```python
from build123d import *

# Parameters (mm, degrees)
SKETCH2_R           = 4
CUT_EXTRUDE1_DEPTH  = 0.5
SKETCH3_R           = 2.2
BOSS_EXTRUDE1_DEPTH = 0.5
SKETCH4_R           = 1.55
CUT_EXTRUDE2_DEPTH  = 16.305227865
CHAMFER1_SIZE       = 0.25


with BuildPart() as part:
    # Sketch1 → Revolve1 (revolve)
    with BuildSketch(Plane.XY, mode=Mode.PRIVATE) as revolve1_sk:
        Polygon((0, 0), (-9, 0), (-9, 1), (-6, 1), (-6, 7.5), (-9, 7.5), (-9, 8.5), (0, 8.5), align=None)
    revolve(revolve1_sk.sketch.rotate(Axis((0, 8.5, 0), (0, -1, 0)), 270), axis=Axis((0, 8.5, 0), (0, -1, 0)))

    # Sketch2 → Cut-Extrude1 (cut)
    with BuildSketch(Plane.XZ):
        with Locations(Location((0, 0, 0), (0, 0, 270))):
            Circle(SKETCH2_R)
    cut_extrude1 = extrude(amount=-CUT_EXTRUDE1_DEPTH, mode=Mode.SUBTRACT)

    # Sketch3 → Boss-Extrude1 (add)
    with BuildSketch(Plane.XZ.offset(-0.5)):
        with Locations(Location((0, 0, 0), (0, 0, 270))):
            Circle(SKETCH3_R)
    boss_extrude1 = extrude(amount=BOSS_EXTRUDE1_DEPTH)

    # Mirror1: Cut-Extrude1, Boss-Extrude1 across plane
    add(cut_extrude1.mirror(Plane.ZX.offset(4.25)), mode=Mode.SUBTRACT)
    add(boss_extrude1.mirror(Plane.ZX.offset(4.25)))

    # Sketch4 → Cut-Extrude2 (cut, through all)
    with BuildSketch(Plane.XZ):
        with Locations(Location((0, 0, 0), (0, 0, 270))):
            Circle(SKETCH4_R)
    extrude(amount=-CUT_EXTRUDE2_DEPTH, mode=Mode.SUBTRACT)

    # Chamfer1
    chamfer1_edges = [part.edges().sort_by_distance(p)[0] for p in [
        (0, 8.5, -9),
        (0, 7.5, -6),
        (0, 1, -6),
        (0, 0, -9),
    ]]
    chamfer(chamfer1_edges, length=CHAMFER1_SIZE)


solid = part.part
```
Work out the finished part from the listing and answer in its coordinate system (mm). A direction names the side the tool comes from. Coordinates: 2 decimals unless noted, no trailing zeros. Loops run counter-clockwise (first coordinate to the right, second up) from the corner with the lowest first, then second, coordinate; pieces in that order, holes last. Notation, with made-up numbers: M -2,15 L 44,15 A21 ccw 44,20 Z; hole C 48.25,45 d11. An arc over 180 degrees is marked long. Use CSV: the item, a comma, the result in double quotes. Start each with the question number.
(1) Given pin 1 Ø6.5 at (x, z) = (-0.5, -0.5) entering from -Y; pin 2 Ø5 at (y, z) = (2, 7) entering from +X; pin 3 Ø4 at (x, y) = (-3, 2.5) entering from -Z; pin 4 Ø5 at (x, y) = (-1.5, 4) entering from -Z, each flat-ended and moving along its own axis, determine where each tip first touches the part or whether it passes through.
(2) For a pull along Z with two mould halves and no side action, classify faces 1 (the face through (-1.44, 8.5, -0.95)), 2 (the face through (2.18, 8.25, 0.29)), 3 (the face through (-2.703, 7.88, 8.584)) as +Z half, -Z half, draft (parallel to the pull), parting line (faces both ways), or undercut.
(3) Consider line 1 (X direction, y = 8.15, z = 0); line 2 (Y direction, x = 2, z = -8); line 3 (X direction, y = 3.75, z = 0). Determine where each line is inside the solid, lowest interval first.
(4) Find section A-A, the plane y = 2.5. Give the vertices of the cut face in (x, z).
(5) For faces 4 (the face through (1.87, 7.5, 6.13)), 5 (the face through (2, 0, -4)), 6 (the face through (-2, 0.5, -2)), 7 (the face through (-3.905, 8.254, 0.867)), determine the directions among +Z, -Z, +X, -X, +Y, -Y from which every point of the face is accessible in a straight line to the end or side of a thin tool.
Recorded:
1,pin 1,"stops at y = 0"
1,pin 2,"stops at x = 7.67"
1,pin 3,"stops at z = -8.84"
1,pin 4,"stops at z = -6"
2,face 1,"draft"
2,face 2,"undercut"
2,face 3,"parting line"
3,line 1,"x = -9 to -4, -2.2 to -1.55, 1.55 to 2.2, 4 to 9"
3,line 2,"y = 0 to 1, 7.5 to 8.5"
3,line 3,"x = -6 to -1.55, 1.55 to 6"
4,outline,"C 0,0 d12; hole C 0,0 d3.1"
5,face 4,"none"
5,face 5,"+Z, -Z, +X, -X, -Y"
5,face 6,"-Y"
5,face 7,"+Y"
